```python
from build123d import *

# Parameters (mm, degrees)
F5_D      = 7.4
F5_DEPTH  = 2
F5_START  = 2.3628878
F5_TIP    = 2.2231842904
F8_D      = 2
F10_W     = 1.5
F10_H     = 1.7
F11_DEPTH = 1.8
F13_W     = 1.5
F13_H     = 1.5
F14_DEPTH = 12.9


# Not quite as in the source:
# - a fillet or chamfer that OpenCascade refuses, or shapes differently, is made with other operations: its cross-section is extruded or revolved along the edge and cut away or added


with BuildPart() as f1:
    # F0 (on Right) → F1 (revolve)
    with BuildSketch(Plane.YZ):
        Polygon((-2.5, 27.272233048), (-3.5, 27.272233048), (-3.5, 9.072233048), (-6.25, 9.072233048), (-6.25, 8.1851361653), (-4.55, 8.1851361653), (-4.55, 6.4851361653), (-6.25, 6.4851361653), (-6.25, 5.042233048), (-6.25, -10.627766952), (-5, -10.627766952), (-5, 5.042233048), (-2.5, 7.3351361653), align=None)
    revolve(axis=Axis((0, 0, 6.4422870055), (0, 0, -1)))

    # F2: fillet of radius 1.4485281374 on 1 edges, made by hand

    # F2_s1 → F2_t2 (revolve, cut)
    with BuildSketch(Plane.YZ):
        with BuildLine():
            ThreePointArc((-2.5, 27.272233048), (-3.2236363972, 26.7459334429), (-3.5, 25.8948963881))
            Line((-3.5, 25.8948963881), (-3.5, 27.272233048))
            Line((-3.5, 27.272233048), (-2.5, 27.272233048))
        make_face()
    revolve(axis=Axis((0, 0, 27.272233048), (0, 0, -1)), mode=Mode.SUBTRACT)

    # F5
    # its depths count from where the whole tool has entered the part; down to there all is cleared
    with Locations(Plane.YZ.offset(7.4)):
        with Locations((0, 1.622233048)):
            Hole(F5_D / 2, depth=F5_START)
    with Locations(Plane.YZ.offset(7.4).offset(-F5_START)):
        with Locations((0, 1.622233048)):
            Hole(F5_D / 2, depth=F5_DEPTH)
            with Locations((0, 0, -(F5_DEPTH + F5_TIP / 2))):  # 118° drill point
                Cone(0, F5_D / 2, F5_TIP, mode=Mode.SUBTRACT)

    # F8 (through all)
    with Locations(Plane.XZ.offset(7.5)):
        with Locations((0, -8.077766952), (0, -0.127766952)):
            Hole(F8_D / 2)

    # F13 (on Top) → F14 (join)
    with BuildSketch(Plane.XY):
        with Locations((-5.5, 0)):
            Rectangle(F13_W, F13_H)
    extrude(amount=-F14_DEPTH)


with BuildPart() as f11:
    # F10 (on offset) → F11 (new body)
    with BuildSketch(Plane.YZ.offset(-6.27)):
        with Locations((-0.0197449699, -11.4840940437)):
            Rectangle(F10_W, F10_H)
    extrude(amount=F11_DEPTH)


solid = f1.part
```
The model under review builds one solid part; all positions refer to its coordinate system, in mm. A direction names the side the tool comes from. Round coordinates to 2 decimals unless told otherwise and drop trailing zeros. Order: outer loops, then holes, each group sorted by start corner. A loop starts at its lowest first (then second) coordinate and runs counter-clockwise, first axis right, second up.
Item 1: To check wall thickness, follow probe 1 along Z at (x, y) = (5.3, 0); probe 2 along Z at (x, y) = (-5.25, 2); probe 3 along X at (y, z) = (0.25, -4) (3 decimals). State the ranges of each line that lie inside material, in increasing order.
Working result:
probe 1: z = -10.63 to -2.08, 5.32 to 6.49, 8.19 to 9.07
probe 2: z = -10.63 to 6.49, 8.19 to 9.07
probe 3: x = -6.25 to -4.75, 4.994 to 6.245
Item 2: Add section A-A, the plane x = -5.5. State the section outline as (y, z) points.
Working result:
outline: (-2.97, -10.63) - (-0.75, -10.63) - (-0.75, -12.9) - (0.75, -12.9) - (0.75, -10.63) - (2.97, -10.63) - (2.97, 6.49) - (-2.97, 6.49) - close; (-2.97, 8.19) - (2.97, 8.19) - (2.97, 9.07) - (-2.97, 9.07) - close
Item 3: For pin 1 (6.5 mm diameter, centred on x = 0, y = 0, fed in from -Z); pin 2 (2 mm diameter, centred on x = -4, z = -1.5, fed in from +Y); pin 3 (1.8 mm diameter, centred on x = 0, z = -0.13, fed in from -Y) (1 decimal); pin 4 (1.5 mm diameter, centred on y = -1, z = 15.5, fed in from +X), all flat-tipped, find the tip position at first contact; note any pin that passes through.
Working result:
pin 1: stops at z = 6.65
pin 2: stops at y = 5.48
pin 3: passes through
pin 4: stops at x = 3.49
Item 4: Add section B-B, the plane z = -1.5. State the section outline as (x, y) points.
Working result:
outline: (-6.25, -0.75) - (-6.2, -0.75) arc R6.25 ccw to (5.93, -1.99) - (4.59, -1.99) arc R5 cw to (-4.94, -0.75) - (-4.75, -0.75) - (-4.75, 0.75) - (-4.94, 0.75) arc R5 cw to (4.59, 1.99) - (5.93, 1.99) arc R6.25 ccw to (-6.2, 0.75) - (-6.25, 0.75) - close
Item 5: Draft analysis for pull direction Z (two halves, no side actions). For faces 1 (the flat face through (3, 3, 9.072)), 2 (the flat face through (-4.75, 0, -6)), 3 (the cylindrical face through (1, -5.6, -0.1)), state which applies: released by +Z, released by -Z, zero draft, split by the parting line, or undercut.
Working result:
face 1: released by +Z
face 2: zero draft
face 3: undercut
Item 6: Add section C-C, the plane z = 24. State the section outline as (x, y) points, and give its area (3 significant figures).
Working result:
outline: circle Ø7 at (0, 0); hole circle Ø5 at (0, 0)
area: 18.8 mm2
Item 7: Machinability: for faces 4 (the cylindrical face through (1.341, -3.233, 17.366)), 5 (the cylindrical face through (1, 5.6, -0.1)), 6 (the cylindrical face through (4.44, 0.99, 7.32)), 7 (the flat face through (-6, 0, -12.9)), 8 (the cylindrical face through (5.11, 0.48, 5.29)), which of the approach directions +Z, -Z, +X, -X, +Y, -Y give a long, thin tool a straight path to every point of the face, cutting with its end or side? Answer none if there is none.
Working result:
face 4: +Z
face 5: +Y, -Y
face 6: none
face 7: -Z, +X, -X, +Y, -Y
face 8: +X
Item 8: Add section D-D, the plane x = 0. Count the separate pieces of the cut face and the enclosed holes in it, and give its area (3 significant figures).
Working result:
separate pieces: 6
enclosed holes: 0
area: 83.6 mm2
